The listing builds one solid part. Answer for the finished solid, in the listing's coordinates (mm). Coordinates: 2 decimals unless noted, no trailing zeros. Loops run counter-clockwise (first coordinate to the right, second up) from the corner with the lowest first, then second, coordinate; pieces in that order, holes last. Notation, with made-up numbers: (-3, -19) - (39, -19) arc R21 cw to (39, 16) - close; hole circle Ø2 at (-24, -40). An arc over 180 degrees is marked (long way). Return JSON: item names as keys, results as strings. Group by question number.
1. Section C-C (x = -31) is taken. Write down the section's boundary in (y, z), and give its area (3 significant figures).
2. This flat-tipped pin is pushed along its axis until it touches: P1, Ø3, axis at x = 30.5, z = 2, coming from the +Y side. Where does it stop, or does it pass through?
3. Section B-B (y = -26.5) is taken. Write down the section's boundary in (x, z), and give its area (3 significant figures).
4. The mould has two halves that part along Y. Classify faces 1 (the face through (-29.1, -15, 2)), 2 (the face through (1, 0, 2)), 3 (the face through (-1, -24, 0)): pulls with the +Y half, pulls with the -Y half, needs draft (parallel to the pull), parting line crosses it, or undercut.
5. Section D-D (y = -20) is taken. Write down the section's boundary in (x, z) (3 decimals), and give its area (3 significant figures).
6. Find the intervals of material crossed by line 1 along Y through (x, z) = (15, 3.2) (3 decimals); line 2 along Y through (x, z) = (-46.5, 2.75); line 3 along Y through (x, z) = (0, 3.2) (3 decimals), in increasing order.
7. Section A-A (x = 40.5) is taken. Write down the section's boundary in (y, z), and give its area (3 significant figures).
Autodesk Inventor part; units mm, degrees
ref_plane "YZ Plane" through (0, 0, 0) normal (1, 0, 0) x (0, 1, 0)
ref_plane "XZ Plane" through (0, 0, 0) normal (0, 1, 0) x (-1, 0, 0)
ref_plane "XY Plane" through (0, 0, 0) normal (0, 0, 1) x (1, 0, 0)
sketch "Sketch1" plane through (0, 0, 0) normal (0, 0, 1) x (1, 0, 0)
  line L0 (60, 0) -> (-60, 0)
  line L1 (-60, 0) -> (-60, -40)
  line L2 (-60, -40) -> (60, -40)
  line L3 (60, -40) -> (60, 0)
  line L4 (46.9, -8) -> (38.1, -8)
  line L5 (38.1, -8) -> (38.1, -32)
  line L6 (38.1, -32) -> (46.9, -32)
  line L7 (46.9, -32) -> (46.9, -8)
  line L8 (46.9, -8) -> (46.9, 0) construction
  line L9 (46.9, -32) -> (46.9, -40) construction
  line L10 (0, 0) -> (5.0949, 0) construction
  line L11 (-46.9, -8) -> (-38.1, -8)
  line L12 (-38.1, -8) -> (-38.1, -32)
  line L13 (-38.1, -32) -> (-46.9, -32)
  line L14 (-46.9, -32) -> (-46.9, -8)
  line L15 (-42.5, -23.6928) -> (-38.1, -23.6928) construction
  line L16 (-42.5, -23.6928) -> (-46.9, -23.6928) construction
  line L17 (46.9, -20) -> (60, -20) construction
  line L18 (-60, -20) -> (-46.9, -20) construction
  line L19 (51.9, -10.6667) -> (55.9, -10.6667)
  line L20 (55.9, -10.6667) -> (55.9, -18.6667)
  line L21 (55.9, -18.6667) -> (51.9, -18.6667)
  line L22 (51.9, -18.6667) -> (51.9, -10.6667)
  line L23 (51.9, -21.3333) -> (55.9, -21.3333)
  line L24 (55.9, -21.3333) -> (55.9, -29.3333)
  line L25 (55.9, -29.3333) -> (51.9, -29.3333)
  line L26 (51.9, -29.3333) -> (51.9, -21.3333)
  line L27 (51.9, -10.6667) -> (51.9, -8) construction
  line L28 (46.9, -8) -> (51.9, -8) construction
  line L29 (51.9, -18.6667) -> (51.9, -21.3333) construction
  line L30 (51.9, -29.3333) -> (51.9, -32) construction
  line L31 (46.9, -32) -> (51.9, -32) construction
  line L32 (29.1, -10.6667) -> (33.1, -10.6667)
  line L33 (33.1, -10.6667) -> (33.1, -18.6667)
  line L34 (33.1, -18.6667) -> (29.1, -18.6667)
  line L35 (29.1, -18.6667) -> (29.1, -10.6667)
  line L36 (29.1, -21.3333) -> (33.1, -21.3333)
  line L37 (33.1, -21.3333) -> (33.1, -29.3333)
  line L38 (33.1, -29.3333) -> (29.1, -29.3333)
  line L39 (29.1, -29.3333) -> (29.1, -21.3333)
  line L40 (38.1, -8) -> (33.1, -8) construction
  line L41 (33.1, -8) -> (33.1, -10.6667) construction
  line L42 (33.1, -18.6667) -> (33.1, -21.3333) construction
  line L43 (33.1, -29.3333) -> (33.1, -32) construction
  line L44 (33.1, -32) -> (38.1, -32) construction
  line L45 (-33.1, -10.6667) -> (-29.1, -10.6667)
  line L46 (-29.1, -10.6667) -> (-29.1, -18.6667)
  line L47 (-29.1, -18.6667) -> (-33.1, -18.6667)
  line L48 (-33.1, -18.6667) -> (-33.1, -10.6667)
  line L49 (-33.1, -21.3333) -> (-29.1, -21.3333)
  line L50 (-29.1, -21.3333) -> (-29.1, -29.3333)
  line L51 (-29.1, -29.3333) -> (-33.1, -29.3333)
  line L52 (-33.1, -29.3333) -> (-33.1, -21.3333)
  line L53 (-55.9, -29.3333) -> (-51.9, -29.3333)
  line L54 (-51.9, -29.3333) -> (-51.9, -21.3333)
  line L55 (-51.9, -21.3333) -> (-55.9, -21.3333)
  line L56 (-55.9, -21.3333) -> (-55.9, -29.3333)
  line L57 (-51.9, -10.6667) -> (-55.9, -10.6667)
  line L58 (-55.9, -10.6667) -> (-55.9, -18.6667)
  line L59 (-55.9, -18.6667) -> (-51.9, -18.6667)
  line L60 (-51.9, -18.6667) -> (-51.9, -10.6667)
  line L61 (-33.1, -29.3333) -> (-38.1, -29.3333) construction
  line L62 (-51.9, -29.3333) -> (-46.9, -29.3333) construction
  circle A0 centre (15, -30) radius 2.125
  circle A1 centre (15, -10) radius 2.125
  line L63 (15, -10) -> (15, -30) construction
  line L64 (15, -30) -> (15, -40) construction
  line L65 (15, -10) -> (15, 0) construction
  circle A2 centre (0, -20) radius 2.125
  line L66 (0, -20) -> (0, -40) construction
  line L67 (0, -20) -> (0, 0) construction
  dimension "d0" = 120
  dimension "d1" = 40
  dimension "d2" = 8.8
  dimension "d3" = 24
  dimension "d4" = 8.8
  dimension "d5" = 24
  dimension "d6" = 4
  dimension "d7" = 8
  dimension "d8" = 5
  dimension "d11" = 76.2
  dimension "d14" = 4.25
  dimension "d15" = 4.25
  dimension "d16" = 20
  dimension "d17" = 45
  dimension "d18" = 4.25
extrude "Extrusion1" add sketch "Sketch1" along normal blind 5
sketch "Sketch2" plane through (-46.9, -8, 0) normal (0, -1, 0) x (1, 0, 0)
  circle A0 centre (4.4, 11.0737) radius 7.5
  circle A1 centre (89.4, 11.0737) radius 7.5
  point P0 (46.9, 0)
  point P1 (0, 5)
  point P2 (8.8, 5)
  point P3 (85, 5)
  point P4 (93.8, 5)
  dimension "d12" = 15
  dimension "d13" = 15
properties part number "YCartFloor"
The answers:
{
 "1": {"outline": "(-40, 0) - (-29.33, 0) - (-29.33, 5) - (-40, 5) - close; (-21.33, 0) - (-18.67, 0) - (-18.67, 5) - (-21.33, 5) - close; (-10.67, 0) - (0, 0) - (0, 5) - (-10.67, 5) - close", "area": "120 mm2"},
 "2": {"P1": "stops at y = 0"},
 "3": {"outline": "(-60, 0) - (-55.9, 0) - (-55.9, 5) - (-60, 5) - close; (-51.9, 0) - (-46.9, 0) - (-46.9, 5) - (-51.9, 5) - close; (-38.1, 0) - (-33.1, 0) - (-33.1, 5) - (-38.1, 5) - close; (-29.1, 0) - (29.1, 0) - (29.1, 5) - (-29.1, 5) - close; (33.1, 0) - (38.1, 0) - (38.1, 5) - (33.1, 5) - close; (46.9, 0) - (51.9, 0) - (51.9, 5) - (46.9, 5) - close; (55.9, 0) - (60, 0) - (60, 5) - (55.9, 5) - close", "area": "432 mm2"},
 "4": {"face 1": "undercut", "face 2": "pulls with the +Y half", "face 3": "needs draft"},
 "5": {"outline": "(-60, 0) - (-46.9, 0) - (-46.9, 5) - (-60, 5) - close; (-38.1, 0) - (-2.125, 0) - (-2.125, 5) - (-38.1, 5) - close; (2.125, 0) - (38.1, 0) - (38.1, 5) - (2.125, 5) - close; (46.9, 0) - (60, 0) - (60, 5) - (46.9, 5) - close", "area": "491 mm2"},
 "6": {"line 1": "y = -40 to -32.125, -27.875 to -12.125, -7.875 to 0", "line 2": "y = -40 to -32, -8 to 0", "line 3": "y = -40 to -22.125, -17.875 to 0"},
 "7": {"outline": "(-40, 0) - (-32, 0) - (-32, 5) - (-40, 5) - close; (-8, 0) - (0, 0) - (0, 5) - (-8, 5) - close", "area": "80.0 mm2"}
}
